from build123d import *

# Parameters (mm, degrees)
SKETCH1_R           = 2.15265
BOSS_EXTRUDE1_DEPTH = 3.175
CUT_EXTRUDE1_DEPTH  = 55.094397353


with BuildPart() as part:
    # Sketch1 → Boss-Extrude1 (new body)
    with BuildSketch(Plane.XY):
        with BuildLine():
            Line((0, 1.5875), (0, 33.9725))
            ThreePointArc((0, 33.9725), (-0.464967985, 35.095032015), (-1.5875, 35.56))
            Line((-1.5875, 35.56), (-39.0525, 35.56))
            ThreePointArc((-39.0525, 35.56), (-40.175032015, 35.095032015), (-40.64, 33.9725))
            Line((-40.64, 33.9725), (-40.64, 1.5875))
            ThreePointArc((-40.64, 1.5875), (-40.175032015, 0.464967985), (-39.0525, 0))
            Line((-39.0525, 0), (-1.5875, 0))
            ThreePointArc((-1.5875, 0), (-0.464967985, 0.464967985), (0, 1.5875))
        make_face()
        with Locations((-7.62, 21.59)):
            Circle(SKETCH1_R, mode=Mode.SUBTRACT)
        with Locations((-33.02, 21.59)):
            Circle(SKETCH1_R, mode=Mode.SUBTRACT)
    extrude(amount=BOSS_EXTRUDE1_DEPTH)

    # Sketch2 → Cut-Extrude1 (cut, through all)
    with BuildSketch(Plane(origin=(0, 0, 0), x_dir=(-1, 0, 0), z_dir=(0, 0, -1))):
        Polygon((11.91856275, 15.939478953), (6.375346419, 15.939478953), (6.375346419, 1.648374352), (34.567798224, 1.648374352), (34.567798224, 15.939478953), (28.115147964, 15.939478953), (28.115147964, 29.018004982), (11.91856275, 29.018004982), align=None)
    extrude(amount=-CUT_EXTRUDE1_DEPTH, mode=Mode.SUBTRACT)


solid = part.part
The model under review builds one solid part; all positions refer to its coordinate system, in mm. A direction names the side the tool comes from. Give positions to 0.01 mm unless a question says otherwise; leave off trailing zeros. Order: outer loops, then holes, each group sorted by start corner. A loop starts at its lowest first (then second) coordinate and runs counter-clockwise, first axis right, second up. Notation, with made-up numbers: (-1.5, 59) -> (31.5, 59) arc R18 ccw to (31.5, 73) -> close; hole circle Ø8 at (-29.5, -13.75). An arc over 180 degrees is marked (long way). Write item = value, one per line. Start each with the question number.
(1) For pin 1 Ø4 at (x, y) = (-7.62, 21.59) entering from +Z, flat-tipped, find the tip position at first contact; note if it passes through.
(2) Take a section at D-D (z = 2.7). Write out the cut boundary in (x, y) (1 decimal), plus the area to 3 significant figures.
(3) For L1, parallel to Y at x = -16.5, z = 2.5; L2, parallel to X at y = 14, z = 0.7; L3, parallel to Y at x = -33.02, z = 1, list the stretches that pass through material, from the lowest coordinate up. Write a range as from..to.
(4) Take a section at C-C (x = -13). Write out the cut boundary in (y, z) (3 decimals).
(5) Take a section at B-B (y = 21.59). Write out the cut boundary in (x, z) (3 decimals), plus the area to 3 significant figures.
(6) Draft analysis for pull direction X (two halves, no side actions). For faces 1 (the flat face through (-40.64, 18, 2)), 2 (the flat face through (-21, 0, 2)), 3 (the flat face through (-28.115, 22, 2)), state which applies: +X half, -X half, draft (parallel to the pull), parting line (faces both ways), or undercut.
(7) Tool access review of faces 4 (the flat face through (-21, 30, 0)), 5 (the flat face through (-20, 29.018, 2)): name each direction out of +Z, -Z, +X, -X, +Y, -Y from which nothing blocks a thin tool from reaching the whole face with its end or side.
(8) Take a section at A-A (x = -7.62). Write out the cut boundary in (y, z) (3 decimals), plus the area to 3 significant figures.
Returned:
q1.pin_1 = through
q2.outline = (-40.6, 1.6) arc R1.6 ccw to (-39.1, 0) -> (-1.6, 0) arc R1.6 ccw to (0, 1.6) -> (0, 34) arc R1.6 ccw to (-1.6, 35.6) -> (-39.1, 35.6) arc R1.6 ccw to (-40.6, 34) -> close; hole circle Ø4.3 at (-33, 21.6); hole (-34.6, 1.6) -> (-6.4, 1.6) -> (-6.4, 15.9) -> (-11.9, 15.9) -> (-11.9, 29) -> (-28.1, 29) -> (-28.1, 15.9) -> (-34.6, 15.9) -> close; hole circle Ø4.3 at (-7.6, 21.6)
q2.area = 799 mm²
q3.L1 = 0..1.65, 29.02..35.56
q3.L2 = -40.64..-34.57, -6.38..0
q3.L3 = 0..1.65, 15.94..19.44, 23.74..35.56
q4.outline = (0, 0) -> (1.648, 0) -> (1.648, 3.175) -> (0, 3.175) -> close; (29.018, 0) -> (35.56, 0) -> (35.56, 3.175) -> (29.018, 3.175) -> close
q5.outline = (-40.64, 0) -> (-35.173, 0) -> (-35.173, 3.175) -> (-40.64, 3.175) -> close; (-30.867, 0) -> (-28.115, 0) -> (-28.115, 3.175) -> (-30.867, 3.175) -> close; (-11.919, 0) -> (-9.773, 0) -> (-9.773, 3.175) -> (-11.919, 3.175) -> close; (-5.467, 0) -> (0, 0) -> (0, 3.175) -> (-5.467, 3.175) -> close
q5.area = 50.3 mm²
q6.face_1 = -X half
q6.face_2 = draft
q6.face_3 = undercut
q7.face_4 = -Z, +X, -X, +Y, -Y
q7.face_5 = +Z, -Z
q8.outline = (0, 0) -> (1.648, 0) -> (1.648, 3.175) -> (0, 3.175) -> close; (15.939, 0) -> (19.437, 0) -> (19.437, 3.175) -> (15.939, 3.175) -> close; (23.743, 0) -> (35.56, 0) -> (35.56, 3.175) -> (23.743, 3.175) -> close
q8.area = 53.9 mm²
